from build123d import *

# Parameters (mm, degrees)
SKETCH1_W           = 85
SKETCH1_H           = 55
SKETCH1_R           = 2.5
SKETCH1_W_2         = 15
SKETCH1_H_2         = 9.566733068
BOSS_EXTRUDE1_DEPTH = 1.5
FILLET1_R           = 5


with BuildPart() as part:
    # Sketch1 → Boss-Extrude1 (new body)
    with BuildSketch(Plane(origin=(0, 0, 0), x_dir=(1, 0, 0), z_dir=(0, 1, 0))):
        Rectangle(SKETCH1_W, SKETCH1_H)
        with Locations(Location((-35, 0, 0), (0, 0, 270))):
            Circle(SKETCH1_R, mode=Mode.SUBTRACT)
        with Locations(Location((-29.142135624, 14.142135624, 0), (0, 0, 270))):
            Circle(SKETCH1_R, mode=Mode.SUBTRACT)
        with Locations(Location((-15, 20, 0), (0, 0, 270))):
            Circle(SKETCH1_R, mode=Mode.SUBTRACT)
        with Locations(Location((-0.857864376, 14.142135624, 0), (0, 0, 270))):
            Circle(SKETCH1_R, mode=Mode.SUBTRACT)
        with Locations(Location((5, 0, 0), (0, 0, 270))):
            Circle(SKETCH1_R, mode=Mode.SUBTRACT)
        with Locations(Location((-0.857864376, -14.142135624, 0), (0, 0, 270))):
            Circle(SKETCH1_R, mode=Mode.SUBTRACT)
        with Locations(Location((-15, -20, 0), (0, 0, 270))):
            Circle(SKETCH1_R, mode=Mode.SUBTRACT)
        with Locations(Location((-29.142135624, -14.142135624, 0), (0, 0, 270))):
            Circle(SKETCH1_R, mode=Mode.SUBTRACT)
        with Locations((25, -0.216633466)):
            Rectangle(SKETCH1_W_2, SKETCH1_H_2, mode=Mode.SUBTRACT)
    extrude(amount=BOSS_EXTRUDE1_DEPTH)

    # Fillet1
    fillet1_edges = [part.edges().sort_by_distance(p)[0] for p in [
        (-42.5, 0.75, -27.5),
        (42.5, 0.75, -27.5),
        (42.5, 0.75, 27.5),
        (-42.5, 0.75, 27.5),
    ]]
    fillet(fillet1_edges, radius=FILLET1_R)


solid = part.part
Geometry: final body of the model. Coordinates: model frame, mm. Round coordinates to 2 decimals unless told otherwise and drop trailing zeros. Loops run counter-clockwise (first coordinate to the right, second up) from the corner with the lowest first, then second, coordinate; pieces in that order, holes last. Notation, with made-up numbers: M 61,-15 L 73,-15 A18 cw 73,-4 Z; hole C 77,78 d7. An arc over 180 degrees is marked long. Put each result on its own line as item: value. Start each with the question number.
(1) Section query D-D (z = 0). Return loops of the section in (x, y), then the cut area to 3 significant figures.
(2) Section query B-B (z = -18.5). Return loops of the section in (x, y).
(3) Section query C-C (x = -35). Return loops of the section in (y, z).
(4) Material intervals for line 1 along X through (y, z) = (1.1, 14); line 2 along Z through (x, y) = (24.5, 1.05); line 3 along X through (y, z) = (0.3, 20), sorted ascending. Write a range as [from, to].
(5) Draft query along Z for faces 1 (the face through (-1, 0, 0)), 2 (the face through (-41.07, 0.76, 26)), 3 (the face through (7.48, 0.74, -0.33)). Return one class per face: +Z half, -Z half, draft (parallel to the pull), parting line (faces both ways), or undercut.
(6) Section query A-A (x = -15). Return loops of the section in (y, z), then the cut area to 3 significant figures.
Findings below:
1. outline: M -42.5,0 L -37.5,0 L -37.5,1.5 L -42.5,1.5 Z; M -32.5,0 L 2.5,0 L 2.5,1.5 L -32.5,1.5 Z; M 7.5,0 L 17.5,0 L 17.5,1.5 L 7.5,1.5 Z; M 32.5,0 L 42.5,0 L 42.5,1.5 L 32.5,1.5 Z
1. area: 90.0 mm2
2. outline: M -42.5,0 L -17,0 L -17,1.5 L -42.5,1.5 Z; M -13,0 L 42.5,0 L 42.5,1.5 L -13,1.5 Z
3. outline: M 0,-27.5 L 1.5,-27.5 L 1.5,-2.5 L 0,-2.5 Z; M 0,2.5 L 1.5,2.5 L 1.5,27.5 L 0,27.5 Z
4. line 1: x = [-42.5, -31.64], [-26.65, -3.35], [1.64, 42.5]
4. line 2: z = [-27.5, -4.57], [5, 27.5]
4. line 3: x = [-42.5, -17.5], [-12.5, 42.5]
5. face 1: draft
5. face 2: +Z half
5. face 3: undercut
6. outline: M 0,-27.5 L 1.5,-27.5 L 1.5,-22.5 L 0,-22.5 Z; M 0,-17.5 L 1.5,-17.5 L 1.5,17.5 L 0,17.5 Z; M 0,22.5 L 1.5,22.5 L 1.5,27.5 L 0,27.5 Z
6. area: 67.5 mm2
